The listing builds one solid part. Answer for the finished solid, in the listing's coordinates (mm). A direction names the side the tool comes from. Round coordinates to 2 decimals unless told otherwise and drop trailing zeros. Write each loop counter-clockwise with the first axis right and the second up, starting at its lowest first coordinate (ties: lowest second). Pieces come first, ordered by that corner, then holes.
(1) This flat-tipped pin is pushed along its axis until it touches: pin 1 Ø6 at (x, y) = (29, 62.5) entering from +Z. Where does it stop, or does it pass through?
(2) A cutting plane is placed at C-C, the plane y = 142.5. Give the vertices of the cut face in (x, z).
(3) For faces 3 (the face through (96, 96, 0)), 4 (the face through (135, 101, 6)), determine the directions among +Z, -Z, +X, -X, +Y, -Y from which every point of the face is accessible in a straight line to the end or side of a thin tool.
(4) A cutting plane is placed at B-B, the plane z = 24. Give the vertices of the cut face in (x, y), and give its area (3 significant figures).
(5) Find the intervals of material crossed by probe 1 along X at (y, z) = (122, 15.5); probe 2 along Y at (x, z) = (64.5, 15); probe 3 along X at (y, z) = (17, 31.5), in increasing order.
(6) The mould has two halves that part along X. Classify faces 1 (the face through (96, 189, 27)), 2 (the face through (135, 164, 6)): +X half, -X half, draft (parallel to the pull), parting line (faces both ways), or undercut.
(7) A cutting plane is placed at D-D, the plane x = 127. Give the vertices of the cut face in (y, z), and give its area (3 significant figures).
(8) A cutting plane is placed at A-A, the plane x = 20. Give the vertices of the cut face in (y, z), and give its area (3 significant figures).
from build123d import *

# Parameters (mm, degrees)
SKETCH1_W           = 188.999995589
SKETCH1_H           = 188.999995589
BOSS_EXTRUDE1_DEPTH = 54.000001401
BOSS_EXTRUDE2_DEPTH = 2.999998629
BOSS_EXTRUDE3_DEPTH = 2.999998629
BOSS_EXTRUDE4_DEPTH = 2.999998629
BOSS_EXTRUDE5_DEPTH = 2.999998629
SKETCH6_W           = 174.999997486
SKETCH6_H           = 174.999997486
CUT_EXTRUDE1_DEPTH  = 51.000001375
BOSS_EXTRUDE6_DEPTH = 14.000000898
SKETCH8_W           = 40.000014007
SKETCH8_H           = 68.999998271
BOSS_EXTRUDE7_DEPTH = 5.000000354
SKETCH9_W           = 34.000001848
SKETCH9_H           = 63.000008464
CUT_EXTRUDE2_DEPTH  = 5.000000354


with BuildPart() as part:
    # Sketch1 → Boss-Extrude1 (new body)
    with BuildSketch(Plane(origin=(0, 0, 0), x_dir=(-1, 0, 0), z_dir=(0, 0, -1))):
        with Locations((-94.499997795, 94.499997795)):
            Rectangle(SKETCH1_W, SKETCH1_H)
    extrude(amount=-BOSS_EXTRUDE1_DEPTH)

    # Sketch2 → Boss-Extrude2 (add)
    with BuildSketch(Plane.XY.offset(54.000001401)):
        Polygon((3.152705729, 96.469610929), (3.49999941, 96.500001848), (3.847301006, 96.469610929), (4.184044898, 96.379376948), (4.500002135, 96.232049167), (4.785574973, 96.032083035), (5.032091867, 95.785565674), (5.232051015, 95.499992371), (5.379386246, 95.184035599), (5.469620228, 94.847291708), (5.500003695, 94.499990344), (5.469620228, 94.152703881), (5.379386246, 93.815952539), (5.232051015, 93.499995768), (5.032091867, 93.214422464), (4.785574973, 92.967912555), (4.500002135, 92.767946422), (4.184044898, 92.620611191), (3.847301006, 92.530377209), (3.49999941, 92.500001192), (3.152705729, 92.530377209), (2.815961838, 92.620611191), (2.500005066, 92.767946422), (2.214424312, 92.967912555), (1.967914402, 93.214422464), (1.76794827, 93.499995768), (1.620620489, 93.815952539), (1.530386391, 94.152703881), (1.500003156, 94.499990344), (1.530386391, 94.847291708), (1.620620489, 95.184035599), (1.76794827, 95.499992371), (1.967914402, 95.785565674), (2.214424312, 96.032083035), (2.500005066, 96.232049167), (2.815961838, 96.379376948), align=None)
    extrude(amount=BOSS_EXTRUDE2_DEPTH)

    # Sketch3 → Boss-Extrude3 (add)
    with BuildSketch(Plane.XY.offset(54.000001401)):
        Polygon((96.032090485, 184.214413166), (95.785573125, 183.967918158), (95.499999821, 183.767944574), (95.18404305, 183.620601892), (94.847299159, 183.530375361), (94.499997795, 183.500006795), (94.152703881, 183.530375361), (93.815967441, 183.620601892), (93.500003219, 183.767944574), (93.214422464, 183.967918158), (92.967912555, 184.214413166), (92.767953873, 184.49999392), (92.620611191, 184.815958142), (92.53038466, 185.152694583), (92.500001192, 185.499995947), (92.53038466, 185.847297311), (92.620611191, 186.184033751), (92.767953873, 186.499997973), (92.967912555, 186.785563827), (93.214422464, 187.032088637), (93.500003219, 187.232047319), (93.815967441, 187.3793751), (94.152703881, 187.469601631), (94.499997795, 187.5), (94.847299159, 187.469601631), (95.18404305, 187.3793751), (95.499999821, 187.232047319), (95.785573125, 187.032088637), (96.032090485, 186.785563827), (96.232056618, 186.499997973), (96.379384398, 186.184033751), (96.46961838, 185.847297311), (96.500001848, 185.499995947), (96.46961838, 185.152694583), (96.379384398, 184.815958142), (96.232056618, 184.49999392), align=None)
    extrude(amount=BOSS_EXTRUDE3_DEPTH)

    # Sketch4 → Boss-Extrude4 (add)
    with BuildSketch(Plane.XY.offset(54.000001401)):
        Polygon((185.847297311, 92.530377209), (185.499995947, 92.500001192), (185.152694583, 92.530377209), (184.815958142, 92.620611191), (184.49999392, 92.767946422), (184.214428067, 92.967912555), (183.967918158, 93.214422464), (183.767959476, 93.499995768), (183.620616794, 93.815952539), (183.530375361, 94.152703881), (183.500006795, 94.499990344), (183.530375361, 94.847291708), (183.620616794, 95.184035599), (183.767959476, 95.499992371), (183.967918158, 95.785565674), (184.214428067, 96.032083035), (184.49999392, 96.232049167), (184.815958142, 96.379376948), (185.152694583, 96.469610929), (185.499995947, 96.500001848), (185.847297311, 96.469610929), (186.184033751, 96.379376948), (186.499997973, 96.232049167), (186.785578728, 96.032083035), (187.032088637, 95.785565674), (187.232062221, 95.499992371), (187.379390001, 95.184035599), (187.469616532, 94.847291708), (187.5, 94.499990344), (187.469616532, 94.152703881), (187.379390001, 93.815952539), (187.232062221, 93.499995768), (187.032088637, 93.214422464), (186.785578728, 92.967912555), (186.499997973, 92.767946422), (186.184033751, 92.620611191), align=None)
    extrude(amount=BOSS_EXTRUDE4_DEPTH)

    # Sketch5 → Boss-Extrude5 (add)
    with BuildSketch(Plane.XY.offset(54.000001401)):
        Polygon((92.967912555, 2.214424312), (92.767953873, 2.499997616), (92.620611191, 2.815954387), (92.53038466, 3.152698278), (92.500001192, 3.49999941), (92.53038466, 3.847293556), (92.620611191, 4.184036981), (92.767953873, 4.499994218), (92.967912555, 4.785574973), (93.214422464, 5.032084882), (93.500003219, 5.232051015), (93.815967441, 5.379378796), (94.152703881, 5.469612777), (94.499997795, 5.499996245), (94.847299159, 5.469612777), (95.18404305, 5.379378796), (95.499999821, 5.232051015), (95.785573125, 5.032084882), (96.032090485, 4.785574973), (96.232056618, 4.499994218), (96.379384398, 4.184036981), (96.46961838, 3.847293556), (96.500001848, 3.49999941), (96.46961838, 3.152698278), (96.379384398, 2.815954387), (96.232056618, 2.499997616), (96.032090485, 2.214424312), (95.785573125, 1.967906952), (95.499999821, 1.76794827), (95.18404305, 1.620613155), (94.847299159, 1.530379057), (94.499997795, 1.499995589), (94.152703881, 1.530379057), (93.815967441, 1.620613155), (93.500003219, 1.76794827), (93.214422464, 1.967906952), align=None)
    extrude(amount=BOSS_EXTRUDE5_DEPTH)

    # Sketch6 → Cut-Extrude1 (cut)
    with BuildSketch(Plane.XY.offset(54.000001401)):
        with Locations((94.499997562, 94.499997562)):
            Rectangle(SKETCH6_W, SKETCH6_H)
    extrude(amount=-CUT_EXTRUDE1_DEPTH, mode=Mode.SUBTRACT)

    # Sketch7 → Boss-Extrude6 (add)
    with BuildSketch(Plane.XY.offset(3.000000026)):
        Polygon((96.136428416, 160.99999845), (46.136427671, 160.99999845), (46.136427671, 108.999997377), (43.136429042, 108.999997377), (43.136429042, 164.00000453), (99.136427045, 164.00000453), (99.136427045, 108.999997377), (96.136428416, 108.999997377), align=None)
    extrude(amount=BOSS_EXTRUDE6_DEPTH)

    # Sketch8 → Boss-Extrude7 (add)
    with BuildSketch(Plane.XY.offset(3.000000026)):
        with Locations((134.927961976, 132.499996573)):
            Rectangle(SKETCH8_W, SKETCH8_H)
    extrude(amount=BOSS_EXTRUDE7_DEPTH)

    # Sketch9 → Cut-Extrude2 (cut)
    with BuildSketch(Plane.XY.offset(8.00000038)):
        with Locations((134.927961975, 132.500000298)):
            Rectangle(SKETCH9_W, SKETCH9_H)
    extrude(amount=-CUT_EXTRUDE2_DEPTH, mode=Mode.SUBTRACT)


solid = part.part
Solutions:
1. pin 1: stops at z = 3
2. outline: (0, 0) - (189, 0) - (189, 54) - (182, 54) - (182, 3) - (154.93, 3) - (154.93, 8) - (151.93, 8) - (151.93, 3) - (117.93, 3) - (117.93, 8) - (114.93, 8) - (114.93, 3) - (99.14, 3) - (99.14, 17) - (96.14, 17) - (96.14, 3) - (46.14, 3) - (46.14, 17) - (43.14, 17) - (43.14, 3) - (7, 3) - (7, 54) - (0, 54) - close
3. face 3: -Z, +X, -X, +Y, -Y
3. face 4: +Z
4. outline: (0, 0) - (189, 0) - (189, 189) - (0, 189) - close; hole (7, 7) - (182, 7) - (182, 182) - (7, 182) - close
4. area: 5,100 mm2
5. probe 1: x = 0 to 7, 43.14 to 46.14, 96.14 to 99.14, 182 to 189
5. probe 2: y = 0 to 7, 161 to 164, 182 to 189
5. probe 3: x = 0 to 7, 182 to 189
6. face 1: draft
6. face 2: undercut
7. outline: (0, 0) - (189, 0) - (189, 54) - (182, 54) - (182, 3) - (167, 3) - (167, 8) - (164, 8) - (164, 3) - (101, 3) - (101, 8) - (98, 8) - (98, 3) - (7, 3) - (7, 54) - (0, 54) - close
7. area: 1,310 mm2
8. outline: (0, 0) - (189, 0) - (189, 54) - (182, 54) - (182, 3) - (7, 3) - (7, 54) - (0, 54) - close
8. area: 1,280 mm2
